CAD build for the part. Positions are in the model's coordinates, mm. A direction names the side the tool comes from. Give positions to 0.01 mm unless a question says otherwise; leave off trailing zeros. Write each loop counter-clockwise with the first axis right and the second up, starting at its lowest first coordinate (ties: lowest second). Pieces come first, ordered by that corner, then holes. Notation, with made-up numbers: (-21.75, 86) -> (-6.75, 86) arc R25 cw to (-6.75, 102) -> close; hole circle Ø2 at (-35.5, 72). An arc over 180 degrees is marked (long way). Answer as a JSON object with one key per item and string values.
```python
from build123d import *

# Parameters (mm, degrees)
SIX_INTEGRAL_DRY_MAGNET_WELL_ISLANDS_SKE_R     = 7.5
SIX_INTEGRAL_DRY_MAGNET_WELL_ISLANDS_DEPTH     = 4
INTEGRAL_6MM_WIDE_CHANNEL_DIVIDER_SKETCH_W     = 6
INTEGRAL_6MM_WIDE_CHANNEL_DIVIDER_SKETCH_H     = 21
INTEGRAL_6MM_WIDE_CHANNEL_DIVIDER_DEPTH        = 4
SEVEN_DRY_BLIND_MAGNET_WELLS_DEPTH4P5_SK_R     = 6.15
SEVEN_DRY_BLIND_MAGNET_WELLS_DEPTH4P5_SK_R_2   = 4.15
SEVEN_DRY_BLIND_MAGNET_WELLS_DEPTH4P5_DEPTH    = 4.5
CENTER_WELL_ID14X1P5_FACE_GLAND_SKETCH_R       = 8.75
CENTER_WELL_ID14X1P5_FACE_GLAND_SKETCH_R_2     = 6.75
CENTER_WELL_ID14X1P5_FACE_GLAND_DEPTH          = 1.15
OUTER_DRY_WELL_FACE_GLAND_1_SKETCH_R           = 6.75
OUTER_DRY_WELL_FACE_GLAND_1_SKETCH_R_2         = 4.75
OUTER_DRY_WELL_FACE_GLAND_1_DEPTH              = 1.15
OUTER_DRY_WELL_FACE_GLAND_2_SKETCH_R           = 6.75
OUTER_DRY_WELL_FACE_GLAND_2_SKETCH_R_2         = 4.75
OUTER_DRY_WELL_FACE_GLAND_2_DEPTH              = 1.15
OUTER_DRY_WELL_FACE_GLAND_3_SKETCH_R           = 6.75
OUTER_DRY_WELL_FACE_GLAND_3_SKETCH_R_2         = 4.75
OUTER_DRY_WELL_FACE_GLAND_3_DEPTH              = 1.15
OUTER_DRY_WELL_FACE_GLAND_4_SKETCH_R           = 6.75
OUTER_DRY_WELL_FACE_GLAND_4_SKETCH_R_2         = 4.75
OUTER_DRY_WELL_FACE_GLAND_4_DEPTH              = 1.15
OUTER_DRY_WELL_FACE_GLAND_5_SKETCH_R           = 6.75
OUTER_DRY_WELL_FACE_GLAND_5_SKETCH_R_2         = 4.75
OUTER_DRY_WELL_FACE_GLAND_5_DEPTH              = 1.15
OUTER_DRY_WELL_FACE_GLAND_6_SKETCH_R           = 6.75
OUTER_DRY_WELL_FACE_GLAND_6_SKETCH_R_2         = 4.75
OUTER_DRY_WELL_FACE_GLAND_6_DEPTH              = 1.15
PERIMETER_ID62X2_FACE_GLAND_SKETCH_R           = 33.3
PERIMETER_ID62X2_FACE_GLAND_SKETCH_R_2         = 30.7
PERIMETER_ID62X2_FACE_GLAND_DEPTH              = 1.5
SIX_REAR_M3_PILOT_POCKETS_PCD74_SKETCH_R       = 1.25
SIX_REAR_M3_PILOT_POCKETS_PCD74_DEPTH          = 4
THREE_START                                    = 4
THREE_INDEPENDENT_TARGET_CLAMP_PILOT_2_R       = 1.25
THREE_INDEPENDENT_TARGET_CLAMP_PILOTS_PC_DEPTH = 3


with BuildPart() as part:
    # Axial blank profile → Native revolved blank (revolve)
    with BuildSketch(Plane.XY, mode=Mode.PRIVATE) as native_revolved_blank_sk:
        Polygon((0, 0), (7, 0), (7, 41), (0, 41), (0, 29), (4, 29), (4, 10), (0, 10), align=None)
    revolve(native_revolved_blank_sk.sketch.rotate(Axis((-60, 0, 0), (1, 0, 0)), 90), axis=Axis((-60, 0, 0), (1, 0, 0)))

    # Six integral dry magnet-well islands sketch → Six integral dry magnet-well islands (add)
    with BuildSketch(Plane(origin=(0, 0, 0), x_dir=(0, 0, -1), z_dir=(1, 0, 0))):
        with Locations((0, 20)):
            Circle(SIX_INTEGRAL_DRY_MAGNET_WELL_ISLANDS_SKE_R)
        with Locations((-17.320508076, 10)):
            Circle(SIX_INTEGRAL_DRY_MAGNET_WELL_ISLANDS_SKE_R)
        with Locations((-17.320508076, -10)):
            Circle(SIX_INTEGRAL_DRY_MAGNET_WELL_ISLANDS_SKE_R)
        with Locations((0, -20)):
            Circle(SIX_INTEGRAL_DRY_MAGNET_WELL_ISLANDS_SKE_R)
        with Locations((17.320508076, -10)):
            Circle(SIX_INTEGRAL_DRY_MAGNET_WELL_ISLANDS_SKE_R)
        with Locations((17.320508076, 10)):
            Circle(SIX_INTEGRAL_DRY_MAGNET_WELL_ISLANDS_SKE_R)
    extrude(amount=SIX_INTEGRAL_DRY_MAGNET_WELL_ISLANDS_DEPTH)

    # Integral 6mm-wide channel divider sketch → Integral 6mm-wide channel divider (add)
    with BuildSketch(Plane(origin=(0, 0, 0), x_dir=(0, 0, -1), z_dir=(1, 0, 0))):
        with Locations((0, 19.5)):
            Rectangle(INTEGRAL_6MM_WIDE_CHANNEL_DIVIDER_SKETCH_W, INTEGRAL_6MM_WIDE_CHANNEL_DIVIDER_SKETCH_H)
    extrude(amount=INTEGRAL_6MM_WIDE_CHANNEL_DIVIDER_DEPTH)

    # Seven dry blind magnet wells depth4p5 sketch → Seven dry blind magnet wells depth4p5 (cut)
    with BuildSketch(Plane(origin=(0, 0, 0), x_dir=(0, 0, -1), z_dir=(1, 0, 0))):
        Circle(SEVEN_DRY_BLIND_MAGNET_WELLS_DEPTH4P5_SK_R)
        with Locations((0, 20)):
            Circle(SEVEN_DRY_BLIND_MAGNET_WELLS_DEPTH4P5_SK_R_2)
        with Locations((-17.320508076, 10)):
            Circle(SEVEN_DRY_BLIND_MAGNET_WELLS_DEPTH4P5_SK_R_2)
        with Locations((-17.320508076, -10)):
            Circle(SEVEN_DRY_BLIND_MAGNET_WELLS_DEPTH4P5_SK_R_2)
        with Locations((0, -20)):
            Circle(SEVEN_DRY_BLIND_MAGNET_WELLS_DEPTH4P5_SK_R_2)
        with Locations((17.320508076, -10)):
            Circle(SEVEN_DRY_BLIND_MAGNET_WELLS_DEPTH4P5_SK_R_2)
        with Locations((17.320508076, 10)):
            Circle(SEVEN_DRY_BLIND_MAGNET_WELLS_DEPTH4P5_SK_R_2)
    extrude(amount=SEVEN_DRY_BLIND_MAGNET_WELLS_DEPTH4P5_DEPTH, mode=Mode.SUBTRACT)

    # Center-well ID14x1p5 face gland sketch → Center-well ID14x1p5 face gland (cut)
    with BuildSketch(Plane(origin=(0, 0, 0), x_dir=(0, 0, -1), z_dir=(1, 0, 0))):
        Circle(CENTER_WELL_ID14X1P5_FACE_GLAND_SKETCH_R)
        Circle(CENTER_WELL_ID14X1P5_FACE_GLAND_SKETCH_R_2, mode=Mode.SUBTRACT)
    extrude(amount=CENTER_WELL_ID14X1P5_FACE_GLAND_DEPTH, mode=Mode.SUBTRACT)

    # Outer dry-well face gland 1 sketch → Outer dry-well face gland 1 (cut)
    with BuildSketch(Plane(origin=(0, 0, 0), x_dir=(0, 0, -1), z_dir=(1, 0, 0))):
        with Locations((0, 20)):
            Circle(OUTER_DRY_WELL_FACE_GLAND_1_SKETCH_R)
        with Locations((0, 20)):
            Circle(OUTER_DRY_WELL_FACE_GLAND_1_SKETCH_R_2, mode=Mode.SUBTRACT)
    extrude(amount=OUTER_DRY_WELL_FACE_GLAND_1_DEPTH, mode=Mode.SUBTRACT)

    # Outer dry-well face gland 2 sketch → Outer dry-well face gland 2 (cut)
    with BuildSketch(Plane(origin=(0, 0, 0), x_dir=(0, 0, -1), z_dir=(1, 0, 0))):
        with Locations((-17.320508076, 10)):
            Circle(OUTER_DRY_WELL_FACE_GLAND_2_SKETCH_R)
        with Locations((-17.320508076, 10)):
            Circle(OUTER_DRY_WELL_FACE_GLAND_2_SKETCH_R_2, mode=Mode.SUBTRACT)
    extrude(amount=OUTER_DRY_WELL_FACE_GLAND_2_DEPTH, mode=Mode.SUBTRACT)

    # Outer dry-well face gland 3 sketch → Outer dry-well face gland 3 (cut)
    with BuildSketch(Plane(origin=(0, 0, 0), x_dir=(0, 0, -1), z_dir=(1, 0, 0))):
        with Locations((-17.320508076, -10)):
            Circle(OUTER_DRY_WELL_FACE_GLAND_3_SKETCH_R)
        with Locations((-17.320508076, -10)):
            Circle(OUTER_DRY_WELL_FACE_GLAND_3_SKETCH_R_2, mode=Mode.SUBTRACT)
    extrude(amount=OUTER_DRY_WELL_FACE_GLAND_3_DEPTH, mode=Mode.SUBTRACT)

    # Outer dry-well face gland 4 sketch → Outer dry-well face gland 4 (cut)
    with BuildSketch(Plane(origin=(0, 0, 0), x_dir=(0, 0, -1), z_dir=(1, 0, 0))):
        with Locations((0, -20)):
            Circle(OUTER_DRY_WELL_FACE_GLAND_4_SKETCH_R)
        with Locations((0, -20)):
            Circle(OUTER_DRY_WELL_FACE_GLAND_4_SKETCH_R_2, mode=Mode.SUBTRACT)
    extrude(amount=OUTER_DRY_WELL_FACE_GLAND_4_DEPTH, mode=Mode.SUBTRACT)

    # Outer dry-well face gland 5 sketch → Outer dry-well face gland 5 (cut)
    with BuildSketch(Plane(origin=(0, 0, 0), x_dir=(0, 0, -1), z_dir=(1, 0, 0))):
        with Locations((17.320508076, -10)):
            Circle(OUTER_DRY_WELL_FACE_GLAND_5_SKETCH_R)
        with Locations((17.320508076, -10)):
            Circle(OUTER_DRY_WELL_FACE_GLAND_5_SKETCH_R_2, mode=Mode.SUBTRACT)
    extrude(amount=OUTER_DRY_WELL_FACE_GLAND_5_DEPTH, mode=Mode.SUBTRACT)

    # Outer dry-well face gland 6 sketch → Outer dry-well face gland 6 (cut)
    with BuildSketch(Plane(origin=(0, 0, 0), x_dir=(0, 0, -1), z_dir=(1, 0, 0))):
        with Locations((17.320508076, 10)):
            Circle(OUTER_DRY_WELL_FACE_GLAND_6_SKETCH_R)
        with Locations((17.320508076, 10)):
            Circle(OUTER_DRY_WELL_FACE_GLAND_6_SKETCH_R_2, mode=Mode.SUBTRACT)
    extrude(amount=OUTER_DRY_WELL_FACE_GLAND_6_DEPTH, mode=Mode.SUBTRACT)

    # Perimeter ID62x2 face gland sketch → Perimeter ID62x2 face gland (cut)
    with BuildSketch(Plane(origin=(0, 0, 0), x_dir=(0, 0, -1), z_dir=(1, 0, 0))):
        Circle(PERIMETER_ID62X2_FACE_GLAND_SKETCH_R)
        Circle(PERIMETER_ID62X2_FACE_GLAND_SKETCH_R_2, mode=Mode.SUBTRACT)
    extrude(amount=PERIMETER_ID62X2_FACE_GLAND_DEPTH, mode=Mode.SUBTRACT)

    # Six rear M3 pilot pockets PCD74 sketch → Six rear M3 pilot pockets PCD74 (cut)
    with BuildSketch(Plane(origin=(0, 0, 0), x_dir=(0, 0, -1), z_dir=(1, 0, 0))):
        with Locations((0, 37)):
            Circle(SIX_REAR_M3_PILOT_POCKETS_PCD74_SKETCH_R)
        with Locations((-32.04293994, 18.5)):
            Circle(SIX_REAR_M3_PILOT_POCKETS_PCD74_SKETCH_R)
        with Locations((-32.04293994, -18.5)):
            Circle(SIX_REAR_M3_PILOT_POCKETS_PCD74_SKETCH_R)
        with Locations((0, -37)):
            Circle(SIX_REAR_M3_PILOT_POCKETS_PCD74_SKETCH_R)
        with Locations((32.04293994, -18.5)):
            Circle(SIX_REAR_M3_PILOT_POCKETS_PCD74_SKETCH_R)
        with Locations((32.04293994, 18.5)):
            Circle(SIX_REAR_M3_PILOT_POCKETS_PCD74_SKETCH_R)
    extrude(amount=SIX_REAR_M3_PILOT_POCKETS_PCD74_DEPTH, mode=Mode.SUBTRACT)

    # Three independent target-clamp pilot 2 → Three independent target-clamp pilots PC (cut)
    with BuildSketch(Plane(origin=(0, 0, 0), x_dir=(0, 0, -1), z_dir=(1, 0, 0)).offset(THREE_START)):
        with Locations((-18.5, 32.04293994)):
            Circle(THREE_INDEPENDENT_TARGET_CLAMP_PILOT_2_R)
        with Locations((-18.5, -32.04293994)):
            Circle(THREE_INDEPENDENT_TARGET_CLAMP_PILOT_2_R)
        with Locations((37, 0)):
            Circle(THREE_INDEPENDENT_TARGET_CLAMP_PILOT_2_R)
    extrude(amount=THREE_INDEPENDENT_TARGET_CLAMP_PILOTS_PC_DEPTH, mode=Mode.SUBTRACT)


solid = part.part
```
1) Slice it at B-B (z = -37). List the corners of the cut face in (x, y), then the cut area to 3 significant figures.
Model answer:
{"outline": "(0, -17.66) -> (7, -17.66) -> (7, -1.25) -> (4, -1.25) -> (4, 1.25) -> (7, 1.25) -> (7, 17.66) -> (0, 17.66) -> close", "area": "240 mm2"}
2) Wall check: probe 1 along Z at (x, y) = (3, 25); probe 2 along Z at (x, y) = (2.25, 5); probe 3 along X at (y, z) = (0.5, 21). Give the ranges that are in metal, low to high.
Model answer:
{"probe 1": "z = -32.5 to -14.7, -5.59 to 5.59, 14.7 to 32.5", "probe 2": "z = -40.69 to -28.57, -22.91 to -11.73, -8.66 to -3.58, 3.58 to 8.66, 11.73 to 22.91, 28.57 to 40.69", "probe 3": "x = 4 to 7"}
3) Pin check, flat tips, straight feed: pin 1 (1.5 mm diameter, centred on x = 4.5, y = 7.5, fed in from -Z); pin 2 (11 mm diameter, centred on y = -11, z = 15, fed in from -X); pin 3 (2.5 mm diameter, centred on y = 22, z = 2, fed in from -X); pin 4 (3 mm diameter, centred on x = 3.5, y = 12, fed in from +Z). Stop position of each tip, or through.
Model answer:
{"pin 1": "stops at z = -40.44", "pin 2": "stops at x = 0", "pin 3": "stops at x = 4.5", "pin 4": "stops at z = 39.63"}
4) 3-axis set-ups, long thin cutter, end or side, ignore diameter. For faces 3 (the cylindrical face through (0.567, 5.786, -19.512)), 4 (the cylindrical face through (5.479, -32.522, 17.345)): which of +Z, -Z, +X, -X, +Y, -Y reach the whole face in a straight line?
Model answer:
{"face 3": "-X", "face 4": "+X"}
5) Slice it at A-A (y = -37). List the corners of the cut face in (x, z), then the cut area to 3 significant figures.
Model answer:
{"outline": "(0, -17.66) -> (7, -17.66) -> (7, 17.66) -> (0, 17.66) -> (0, 1.25) -> (4, 1.25) -> (4, -1.25) -> (0, -1.25) -> close", "area": "237 mm2"}
6) Mould opens along Z. For faces 1 (the flat face through (7, -1, 1)), 2 (the cylindrical face through (1.97, -18.98, 30.89)) say: released by +Z, released by -Z, zero draft, split by the parting line, or undercut.
Model answer:
{"face 1": "zero draft", "face 2": "undercut"}
7) Slice it at C-C (x = 6). List the corners of the cut face in (y, z).
Model answer:
{"outline": "circle Ø82 at (0, 0); hole circle Ø2.5 at (-32.04, 18.5); hole circle Ø2.5 at (0, -37); hole circle Ø2.5 at (32.04, 18.5)"}
